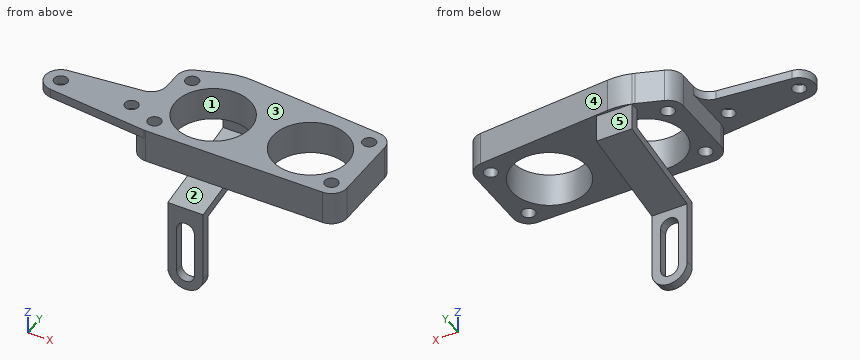
from build123d import *

# Parameters (mm, degrees)
SKETCH1_R           = 8.5
SKETCH1_R_2         = 1.5
BOSS_EXTRUDE1_DEPTH = 7.5
BOSS_EXTRUDE2_START = -2
SKETCH2_R           = 1.5
BOSS_EXTRUDE2_DEPTH = 2
EXTRUDE_THIN1_DEPTH = 4
BOSS_EXTRUDE3_START = -7.5
BOSS_EXTRUDE3_DEPTH = 7.5
CUT_EXTRUDE1_DEPTH  = 10
FILLET1_R           = 4


with BuildPart() as part:
    # Sketch1 → Boss-Extrude1 (new body)
    with BuildSketch(Plane.XY):
        with BuildLine():
            Line((-12.5, -7.5), (-12.5, 7.5))
            ThreePointArc((-12.5, 7.5), (-11.474873734, 9.974873734), (-9, 11))
            Line((-9, 11), (31, 11))
            ThreePointArc((31, 11), (33.474873734, 9.974873734), (34.5, 7.5))
            Line((34.5, 7.5), (34.5, -7.5))
            ThreePointArc((34.5, -7.5), (33.474873734, -9.974873734), (31, -11))
            Line((31, -11), (-9, -11))
            ThreePointArc((-9, -11), (-11.474873734, -9.974873734), (-12.5, -7.5))
        make_face()
        Circle(SKETCH1_R, mode=Mode.SUBTRACT)
        with Locations((22, 0)):
            Circle(SKETCH1_R, mode=Mode.SUBTRACT)
        with Locations((-9, 7.5)):
            Circle(SKETCH1_R_2, mode=Mode.SUBTRACT)
        with Locations((31, 7.5)):
            Circle(SKETCH1_R_2, mode=Mode.SUBTRACT)
        with Locations((31, -7.5)):
            Circle(SKETCH1_R_2, mode=Mode.SUBTRACT)
        with Locations((-9, -7.5)):
            Circle(SKETCH1_R_2, mode=Mode.SUBTRACT)
    extrude(amount=BOSS_EXTRUDE1_DEPTH)

    # Sketch2 → Boss-Extrude2 (add)
    with BuildSketch(Plane.XY.offset(7.5).offset(BOSS_EXTRUDE2_START)):
        with BuildLine():
            ThreePointArc((-12.5, 3.506965576), (-13.399757461, 1.164159836), (-15.636422136, 0.025900921))
            Line((-15.636422136, 0.025900921), (-31.863577864, -1.668935344))
            ThreePointArc((-31.863577864, -1.668935344), (-35, -5.15), (-31.863577864, -8.631064656))
            Line((-31.863577864, -8.631064656), (-9.363577864, -10.981064656))
            ThreePointArc((-9.363577864, -10.981064656), (-11.600242539, -9.842805741), (-12.5, -7.5))
            Line((-12.5, -7.5), (-12.5, 3.506965576))
        make_face()
        with Locations((-31.5, -5.15)):
            Circle(SKETCH2_R, mode=Mode.SUBTRACT)
        with Locations((-15.5, -5.15)):
            Circle(SKETCH2_R, mode=Mode.SUBTRACT)
    extrude(amount=BOSS_EXTRUDE2_DEPTH)

    # Sketch3 → Extrude-Thin1 (add, symmetric)
    with BuildSketch(Plane(origin=(0, 0, 0), x_dir=(0, 0, -1), z_dir=(1, 0, 0))):
        Polygon((-7.5, 11), (4.5, 11), (8.379193576, -11), (28.379193576, -11), (28.379193576, -9), (10.057392838, -9), (6.178199262, 13), (-7.5, 13), align=None)
    extrude(amount=EXTRUDE_THIN1_DEPTH, both=True)

    # Sketch4 → Boss-Extrude3 (add)
    with BuildSketch(Plane.XY.offset(7.5).offset(BOSS_EXTRUDE3_START)):
        with BuildLine():
            Line((-4.599183693, 12.800293331), (-10.183485485, 10.793836988))
            ThreePointArc((-10.183485485, 10.793836988), (-9.600654035, 10.948074061), (-9, 11))
            Line((-9, 11), (-4, 11))
            Line((-4, 11), (-4, 13))
            ThreePointArc((-4, 13), (-4.300751183, 12.903625044), (-4.599183693, 12.800293331))
        make_face()
        with BuildLine():
            ThreePointArc((1.153263837, 13.552489901), (-1.449926884, 13.523968058), (-4, 13))
            Line((-4, 13), (4, 13))
            Line((4, 13), (4, 11))
            Line((4, 11), (31, 11))
            ThreePointArc((31, 11), (31.148515642, 10.996847595), (31.296763753, 10.987396059))
            Line((31.296763753, 10.987396059), (1.153263837, 13.552489901))
        make_face()
    extrude(amount=BOSS_EXTRUDE3_DEPTH)

    # Sketch5 → Cut-Extrude1 (cut)
    with BuildSketch(Plane(origin=(0, -9, 0), x_dir=(1, 0, 0), z_dir=(0, 1, 0))):
        with BuildLine():
            Line((2, 24.379193576), (2, 14.057392838))
            ThreePointArc((2, 14.057392838), (0, 12.057392838), (-2, 14.057392838))
            Line((-2, 14.057392838), (-2, 24.379193576))
            ThreePointArc((-2, 24.379193576), (0, 26.379193576), (2, 24.379193576))
        make_face()
    extrude(amount=-CUT_EXTRUDE1_DEPTH, mode=Mode.SUBTRACT)

    # Fillet1
    fillet1_edges = [part.edges().sort_by_distance(p)[0] for p in [
        (-4, -10, -28.379193576),
        (4, -10, -28.379193576),
    ]]
    fillet(fillet1_edges, radius=FILLET1_R - 0.0001)  # a hair under: the kernel refuses the full size


solid = part.part
Part model, mm, in its own coordinate system. Face numbers are marked on the shaded views. A direction names the side the tool comes from. Coordinates: 2 decimals unless noted, no trailing zeros. Write each loop counter-clockwise with the first axis right and the second up, starting at its lowest first coordinate (ties: lowest second). Pieces come first, ordered by that corner, then holes. Notation, with made-up numbers: (56.25, 55.25) - (71.25, 55.25) arc R17 ccw to (71.25, 64.25) - close; hole circle Ø1 at (18.25, 72). An arc over 180 degrees is marked (long way). Put each result on its own line as item: value.
1. Probe line 1 along Y through (x, z) = (31, 4); line 2 along Z through (x, y) = (-20, -8.25); line 3 along Y through (x, z) = (-9, 5). List the from-to ranges inside material, lowest first. Write a range as [from, to].
Final values:
line 1: y = [-11, -9], [-6, 6], [9, 11.01]
line 2: z = [5.5, 7.5]
line 3: y = [-11, -9], [-6, 6], [9, 11.22]
2. Band-saw the part on B-B (y = 1.25). Write the cut outline in (x, z), then the cut area to 3 significant figures.
Final values:
outline: (-13.32, 5.5) - (-12.5, 5.5) - (-12.5, 0) - (-8.41, 0) - (-8.41, 7.5) - (-13.32, 7.5) - close; (-4, -8.25) - (4, -8.25) - (4, -6.22) - (-4, -6.22) - close; (8.41, 0) - (13.59, 0) - (13.59, 7.5) - (8.41, 7.5) - close; (30.41, 0) - (34.5, 0) - (34.5, 7.5) - (30.41, 7.5) - close
area: 118 mm²
3. Band-saw the part on D-D (y = 4.5). Write the cut outline in (x, z), then the cut area to 3 significant figures.
Final values:
outline: (-12.5, 0) - (-7.21, 0) - (-7.21, 7.5) - (-12.5, 7.5) - close; (-4, -7.68) - (4, -7.68) - (4, -5.65) - (-4, -5.65) - close; (7.21, 0) - (14.79, 0) - (14.79, 7.5) - (7.21, 7.5) - close; (29.21, 0) - (34.5, 0) - (34.5, 7.5) - (29.21, 7.5) - close
area: 152 mm²
4. Flat gauge pins, fed straight in: pin 1 Ø1.6 at (y, z) = (-9.5, -17) entering from -X; pin 2 Ø1.5 at (y, z) = (-6.5, -10) entering from +X; pin 3 Ø12 at (x, z) = (-4, -2.5) entering from +Y; pin 4 Ø10 at (x, y) = (0, 0) entering from -Z. Where does each tip first touch, or does it go through?
Final values:
pin 1: stops at x = -4
pin 2: stops at x = 4
pin 3: stops at y = 13.6
pin 4: stops at z = -9.35
5. Two-plate mould, pull along Y, no slides. Class the marked faces 1, 2 and 3: +Y half, -Y half, draft (parallel to the pull), parting line (faces both ways), or undercut.
Final values:
face 1: undercut
face 2: -Y half
face 3: draft
6. 3-axis set-ups, long thin cutter, end or side, ignore diameter. For the marked faces 4 and 5: which of +Z, -Z, +X, -X, +Y, -Y reach the whole face in a straight line?
Final values:
face 4: +Z, -Z, +X, +Y
face 5: -Z, +X, -X, +Y
7. Band-saw the part on C-C (z = 2). Write the cut outline in (x, y).
Final values:
outline: (-12.5, -7.5) arc R3.5 ccw to (-9, -11) - (31, -11) arc R3.5 ccw to (34.5, -7.5) - (34.5, 7.5) arc R3.5 ccw to (31.3, 10.99) - (1.15, 13.55) arc R13.6 ccw to (-4, 13) arc R13.6 ccw to (-4.6, 12.8) - (-10.18, 10.79) arc R3.5 ccw to (-12.5, 7.5) - close; hole circle Ø3 at (-9, -7.5); hole circle Ø3 at (-9, 7.5); hole circle Ø17 at (0, 0); hole circle Ø17 at (22, 0); hole circle Ø3 at (31, -7.5); hole circle Ø3 at (31, 7.5)
8. Band-saw the part on A-A (z = -19). Write the cut outline in (x, y), then the cut area to 3 significant figures.
Final values:
outline: (-4, -11) - (-2, -11) - (-2, -9) - (-4, -9) - close; (2, -11) - (4, -11) - (4, -9) - (2, -9) - close
area: 8.00 mm²
